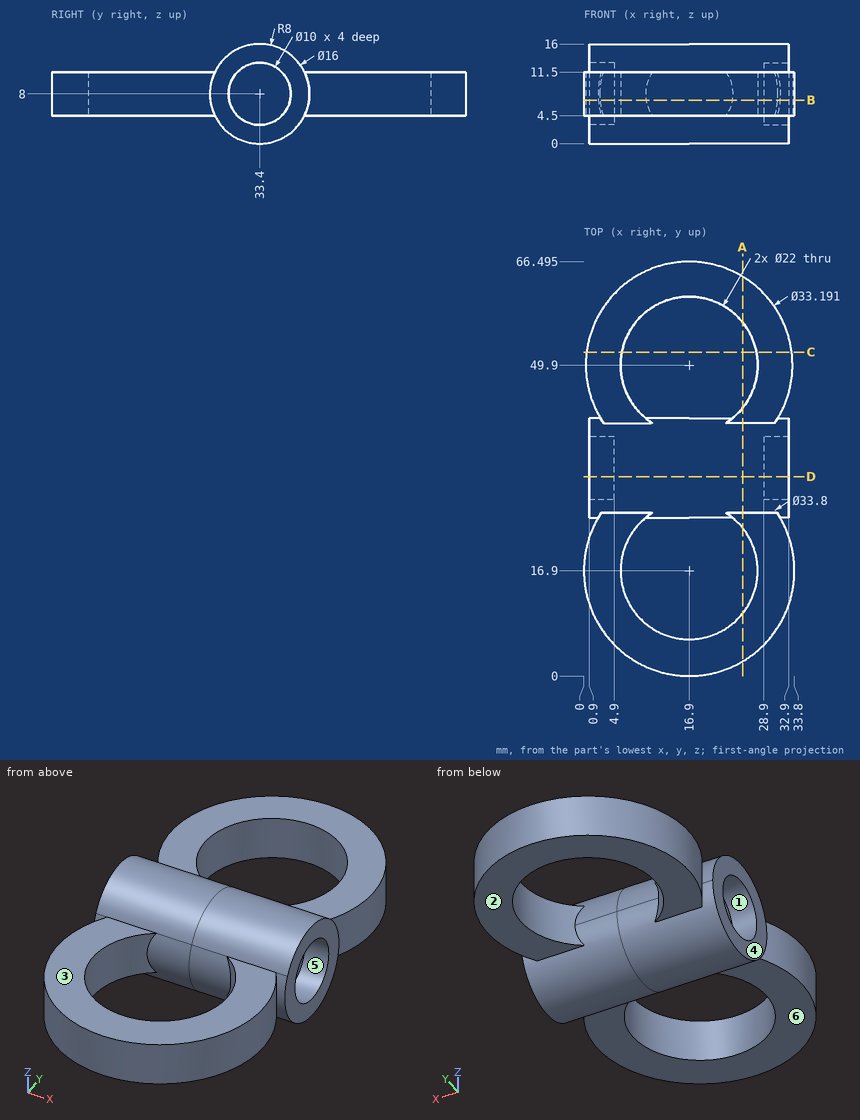
Here's the drawing with two shaded views (mm, measured from the low corner). I have some questions. A direction names the side the tool comes from. Coordinates: 2 decimals unless noted, no trailing zeros. Write each loop counter-clockwise with the first axis right and the second up, starting at its lowest first coordinate (ties: lowest second). Pieces come first, ordered by that corner, then holes. Notation, with made-up numbers: M 70.25,-18.5 L 120.25,-18.5 A5 cw 120.25,-10.5 Z; hole C 16,15 d1. An arc over 180 degrees is marked long. Answer as CSV lines item,"result". Start each with the question number.
1) I want a section at B-B, the plane z = 7. Please give me the cut outline in (x, y) (1 decimal).
2) We'd pull the mould along Z, two halves only. Please class the marked faces 1, 2 and 3: +Z half, -Z half, draft (parallel to the pull), parting line (faces both ways), or undercut.
3) For P1, Ø13, axis at x = 14.5, y = 58.5, coming from the -Z side; P2, Ø3, axis at y = 38, z = 6.5, coming from the +X side; P3, Ø8, axis at y = 34.5, z = 9, coming from the -X side, each with a flat end and sliding along its axis, tell me the tip position at first contact or that it passes through.
4) Please list where these lines run through material, in increasing order: line 1 (Y direction, x = 31.5, z = 11.25) (1 decimal); line 2 (Z direction, x = 2.5, y = 14); line 3 (X direction, y = 43, z = 5.75) (1 decimal). Write a range as from..to.
5) For the marked faces 4, 5 and 6, which set-ups out of +Z, -Z, +X, -X, +Y, -Y let a thin tool reach every point of the face, with its end or its side?
6) I want a section at A-A, the plane x = 25.5. Please give me the cut outline in (y, z), and give its area (3 significant figures).
7) I want a section at C-C, the plane y = 52. Please give me the cut outline in (x, z), and give its area (3 significant figures).
8) I want a section at D-D, the plane y = 32. Please give me the cut outline in (x, z).
Data:
1,outline,"M 0.9,25.5 L 2.3,25.5 A16.9 ccw long 31.5,25.5 L 32.9,25.5 L 32.9,28.5 L 28.9,28.5 L 28.9,38.3 L 32.9,38.3 L 32.9,41.3 L 31.1,41.3 A16.6 ccw long 2.7,41.3 L 0.9,41.3 L 0.9,38.3 L 4.9,38.3 L 4.9,28.5 L 0.9,28.5 Z; hole M 10,25.5 A11 ccw long 23.8,25.5 Z; hole M 10,41.3 L 23.8,41.3 A11 ccw long Z"
2,face 1,"undercut"
2,face 2,"-Z half"
2,face 3,"+Z half"
3,P1,"stops at z = 4.5"
3,P2,"stops at x = 32.9"
3,P3,"stops at x = 0.9"
4,line 1,"y = 8.4..25.4, 26.1..29.6, 37.2..40.7, 42..57.8"
4,line 2,"z = 4.5..11.5"
4,line 3,"x = 1.8..8.3, 25.5..32"
5,face 4,"+Z, -Z, -X"
5,face 5,"+X"
5,face 6,"-Z, +X, -X, -Y"
6,outline,"M 2.35,4.5 L 10.04,4.5 L 10.04,11.5 L 2.35,11.5 Z; M 23.76,4.5 L 26.21,4.5 A8 ccw 40.59,4.5 L 43.04,4.5 L 43.04,11.5 L 40.59,11.5 A8 ccw 26.21,11.5 L 23.76,11.5 Z; M 56.76,4.5 L 64.09,4.5 L 64.09,11.5 L 56.76,11.5 Z"
6,area,"333 mm^2"
7,outline,"M 0.44,4.5 L 6.1,4.5 L 6.1,11.5 L 0.44,11.5 Z; M 27.7,4.5 L 33.36,4.5 L 33.36,11.5 L 27.7,11.5 Z"
7,area,"79.3 mm^2"
8,outline,"M 0.9,0.12 L 32.9,0.12 L 32.9,3.2 L 28.9,3.2 L 28.9,12.8 L 32.9,12.8 L 32.9,15.88 L 0.9,15.88 L 0.9,12.8 L 4.9,12.8 L 4.9,3.2 L 0.9,3.2 Z"
